Here's how the part is built. I have some questions about the finished solid (model axes, mm). Face numbers are marked on the shaded views. A direction names the side the tool comes from. Round coordinates to 2 decimals unless told otherwise and drop trailing zeros. Order: outer loops, then holes, each group sorted by start corner. A loop starts at its lowest first (then second) coordinate and runs counter-clockwise, first axis right, second up. Notation, with made-up numbers: (50.5, 39) -> (59.5, 39) arc R36 ccw to (59.5, 73) -> close; hole circle Ø6 at (83.5, 54.25). An arc over 180 degrees is marked (long way). Use a Markdown table: item, result. Add a question column.
(1) I want a section at D-D, the plane z = -23. Please give me the cut outline in (x, y), then the cut area to 3 significant figures.
(2) If I drill on probe 1 along X at (y, z) = (23.4, -13.5); probe 2 along Z at (x, y) = (15, 23); probe 3 along Z at (x, y) = (-26, 9), over which ranges is the centre line in solid material (lowest first)?
(3) I want a section at C-C, the plane z = -44.5. Please give me the cut outline in (x, y), then the cut area to 3 significant figures.
(4) I'm going to push flat-ended pins straight in: P1, Ø3, axis at x = 32, z = 0, coming from the +Y side; P2, Ø6.5, axis at x = 15.5, z = -45.5, coming from the -Y side; P3, Ø8, axis at y = 11.5, z = 2, coming from the -X side; P4, Ø12, axis at x = -1.5, z = -29, coming from the +Y side. Where does each tip first touch, or does it pass through?
(5) I want a section at B-B, the plane z = -29. Please give me the cut outline in (x, y).
(6) I want a section at A-A, the plane x = 0. Please give me the cut outline in (y, z).
(7) On a 3-axis mill with a long thin cutter (end or side, diameter ignored), from which of +Z, -Z, +X, -X, +Y, -Y can I reach the whole of each face in a straight line? I mean the marked faces 1, 2 and 3. Say none if no direction works.
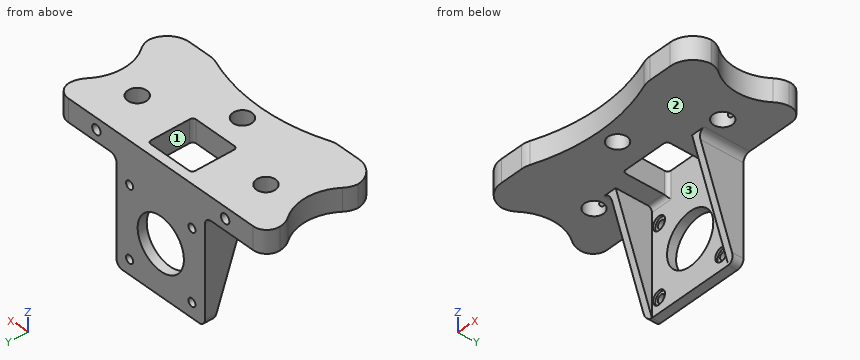
from build123d import *

# Parameters (mm, degrees)
SKETCH1_R           = 4.2
BOSS_EXTRUDE1_DEPTH = 5
FILLET1_R           = 10
FILLET2_R           = 6
SKETCH2_W           = 42
SKETCH2_H           = 46
SKETCH2_R           = 11.5
SKETCH2_R_2         = 1.75
BOSS_EXTRUDE2_DEPTH = 4
CUT_EXTRUDE1_REACH  = 89.139
CUT_EXTRUDE1_START  = -1
SKETCH3_R           = 3
CUT_EXTRUDE2_REACH  = 90.34
SKETCH4_R           = 1.75
SKETCH5_R           = 2.1
CUT_EXTRUDE3_DEPTH  = 4
CHAMFER1_SIZE       = 0.5
BOSS_EXTRUDE3_START = -2
BOSS_EXTRUDE3_DEPTH = 3
FILLET3_R           = 2
FILLET4_R           = 3


with BuildPart() as part:
    # Sketch1 → Boss-Extrude1 (new, symmetric)
    with BuildSketch(Plane.XY):
        with BuildLine():
            Line((-52, 25), (52, 25))
            Line((52, 25), (52, 15.565713714))
            ThreePointArc((52, 15.565713714), (46, 1.282856857), (52, -13))
            Line((52, -13), (52, -25))
            Line((52, -25), (30, -25))
            ThreePointArc((30, -25), (0, -19.161984871), (-30, -25))
            Line((-30, -25), (-52, -25))
            Line((-52, -25), (-52, -13))
            ThreePointArc((-52, -13), (-46, 1.282856857), (-52, 15.565713714))
            Line((-52, 15.565713714), (-52, 25))
        make_face()
        with Locations((0, -11)):
            Circle(SKETCH1_R, mode=Mode.SUBTRACT)
        with Locations((-32, 7)):
            Circle(SKETCH1_R, mode=Mode.SUBTRACT)
        with Locations((32, 7)):
            Circle(SKETCH1_R, mode=Mode.SUBTRACT)
        with BuildLine():
            Line((-9.5, 21), (9.5, 21))
            ThreePointArc((9.5, 21), (10.560660172, 20.560660172), (11, 19.5))
            Line((11, 19.5), (11, 2.5))
            ThreePointArc((11, 2.5), (10.560660172, 1.439339828), (9.5, 1))
            Line((9.5, 1), (-9.5, 1))
            ThreePointArc((-9.5, 1), (-10.560660172, 1.439339828), (-11, 2.5))
            Line((-11, 2.5), (-11, 19.5))
            ThreePointArc((-11, 19.5), (-10.560660172, 20.560660172), (-9.5, 21))
        make_face(mode=Mode.SUBTRACT)
    extrude(amount=BOSS_EXTRUDE1_DEPTH, both=True)

    # Fillet1
    # the kernel refuses this fillet: 10 mm, written as the material it takes off along each edge
    with BuildSketch(Plane(origin=(52, 15.565713714, 14.292857857), x_dir=(-0.6589710561597435, -0.7521682970876347, 0), z_dir=(0, 0, -1))) as fillet1_piece_1:
        with BuildLine():
            CenterArc((3.793793334, 9.971172714), FILLET1_R, 228.778553177, 36.869897646)
            Line((-2.795917228, 2.449489743), (0, 0))
            ThreePointArc((0, 0), (1.517517334, 0.057654573), (3.035034667, 0))
        make_face()
    extrude(amount=28.585715715, mode=Mode.SUBTRACT)
    with BuildSketch(Plane(origin=(52, -13, 14.292857857), x_dir=(0, -1, 0), z_dir=(0, 0, -1)), Plane(origin=(-52, -13, -14.292857857), x_dir=(0, -1, 0), z_dir=(0, 0, 1))) as fillet1_piece_2:
        with BuildLine():
            CenterArc((3.717143143, 10), FILLET1_R, 233.130102354, 36.869897646)
            ThreePointArc((-2.282856857, 2), (-1.103435734, 1.043365942), (0, 0))
            Line((0, 0), (3.717143143, 0))
        make_face()
    extrude(amount=28.585715715, mode=Mode.SUBTRACT)
    with BuildSketch(Plane(origin=(52, -25, 30), x_dir=(-1, 0, 0), z_dir=(0, 0, -1))) as fillet1_piece_3:
        with BuildLine():
            CenterArc((FILLET1_R, FILLET1_R), FILLET1_R, 180, 90)
            Line((0, FILLET1_R), (0, 0))
            Line((0, 0), (FILLET1_R, 0))
        make_face()
    extrude(amount=60, mode=Mode.SUBTRACT)
    with BuildSketch(Plane(origin=(30, -25, 9.716697693), x_dir=(-0.931136532102541, 0.3646707536724787, 0), z_dir=(0, 0, -1))) as fillet1_piece_4:
        with BuildLine():
            CenterArc((1.889951723, 9.999382002), FILLET1_R, 248.612678269, 20.750330625)
            Line((-1.756755813, 0.688016681), (0, 0))
            ThreePointArc((0, 0), (0.889389046, 0.004943983), (1.778778093, 0))
        make_face()
    extrude(amount=19.433395387, mode=Mode.SUBTRACT)
    with BuildSketch(Plane(origin=(-30, -25, 9.716697693), x_dir=(-1, 0, 0), z_dir=(0, 0, -1))) as fillet1_piece_5:
        with BuildLine():
            CenterArc((1.886679077, 10), FILLET1_R, 249.249669375, 20.750330625)
            ThreePointArc((-1.656285265, 0.648668348), (-0.826339706, 0.328937697), (0, 0))
            Line((0, 0), (1.886679077, 0))
        make_face()
    extrude(amount=19.433395387, mode=Mode.SUBTRACT)
    with BuildSketch(Plane(origin=(-52, -25, -30), x_dir=(0, 1, 0), z_dir=(0, 0, 1))) as fillet1_piece_6:
        with BuildLine():
            CenterArc((FILLET1_R, -FILLET1_R), FILLET1_R, 90, 90)
            Line((0, -FILLET1_R), (0, 0))
            Line((0, 0), (FILLET1_R, 0))
        make_face()
    extrude(amount=60, mode=Mode.SUBTRACT)
    with BuildSketch(Plane(origin=(-52, 15.565713714, -14.292857857), x_dir=(0, 1, 0), z_dir=(0, 0, 1))) as fillet1_piece_7:
        with BuildLine():
            CenterArc((3.717143143, -10), FILLET1_R, 90, 36.869897646)
            ThreePointArc((-2.282856857, -2), (-1.103435734, -1.043365942), (0, 0))
            Line((0, 0), (3.717143143, 0))
        make_face()
    extrude(amount=28.585715715, mode=Mode.SUBTRACT)

    # Fillet2
    fillet2_edges = [part.edges().sort_by_distance(p)[0] for p in [
        (52, 25, 0),
        (-52, 25, 0),
    ]]
    fillet(fillet2_edges, radius=FILLET2_R)

    # Sketch2 → Boss-Extrude2 (add)
    with BuildSketch(Plane(origin=(0, 25, -30), x_dir=(-1, 0, 0), z_dir=(0, 1, 0))):
        with Locations((0, 2)):
            Rectangle(SKETCH2_W, SKETCH2_H)
        with Locations(Location((0, 1, 0), (0, 0, 90))):
            Circle(SKETCH2_R, mode=Mode.SUBTRACT)
        with Locations(Location((15.5, 16.5, 0), (0, 0, 90))):
            Circle(SKETCH2_R_2, mode=Mode.SUBTRACT)
        with Locations(Location((-15.5, 16.5, 0), (0, 0, 90))):
            Circle(SKETCH2_R_2, mode=Mode.SUBTRACT)
        with Locations(Location((-15.5, -14.5, 0), (0, 0, 90))):
            Circle(SKETCH2_R_2, mode=Mode.SUBTRACT)
        with Locations(Location((15.5, -14.5, 0), (0, 0, 90))):
            Circle(SKETCH2_R_2, mode=Mode.SUBTRACT)
    extrude(amount=-BOSS_EXTRUDE2_DEPTH)

    # Sketch3 → Cut-Extrude1 (cut, up to next)
    with BuildSketch(Plane.XZ.offset(-21).offset(CUT_EXTRUDE1_START), mode=Mode.PRIVATE) as cut_extrude1_sk1:
        with Locations(Location((-15.5, -44.5, 0), (0, 0, 270))):
            Circle(SKETCH3_R)
    cut_extrude1_tool1 = extrude(cut_extrude1_sk1.sketch, amount=CUT_EXTRUDE1_REACH, mode=Mode.PRIVATE) & part.part
    # Sketch3 → Cut-Extrude1 (cut, up to next)
    with BuildSketch(Plane.XZ.offset(-21).offset(CUT_EXTRUDE1_START), mode=Mode.PRIVATE) as cut_extrude1_sk2:
        with Locations(Location((15.5, -44.5, 0), (0, 0, 270))):
            Circle(SKETCH3_R)
    cut_extrude1_tool2 = extrude(cut_extrude1_sk2.sketch, amount=CUT_EXTRUDE1_REACH, mode=Mode.PRIVATE) & part.part
    # Sketch3 → Cut-Extrude1 (cut, up to next)
    with BuildSketch(Plane.XZ.offset(-21).offset(CUT_EXTRUDE1_START), mode=Mode.PRIVATE) as cut_extrude1_sk3:
        with Locations(Location((15.5, -13.5, 0), (0, 0, 270))):
            Circle(SKETCH3_R)
    cut_extrude1_tool3 = extrude(cut_extrude1_sk3.sketch, amount=CUT_EXTRUDE1_REACH, mode=Mode.PRIVATE) & part.part
    # Sketch3 → Cut-Extrude1 (cut, up to next)
    with BuildSketch(Plane.XZ.offset(-21).offset(CUT_EXTRUDE1_START), mode=Mode.PRIVATE) as cut_extrude1_sk4:
        with Locations(Location((-15.5, -13.5, 0), (0, 0, 270))):
            Circle(SKETCH3_R)
    cut_extrude1_tool4 = extrude(cut_extrude1_sk4.sketch, amount=CUT_EXTRUDE1_REACH, mode=Mode.PRIVATE) & part.part
    add(cut_extrude1_tool1.solids().sort_by_distance((-15.5, 22, -44.5))[0], mode=Mode.SUBTRACT)
    add(cut_extrude1_tool2.solids().sort_by_distance((15.5, 22, -44.5))[0], mode=Mode.SUBTRACT)
    add(cut_extrude1_tool3.solids().sort_by_distance((15.5, 22, -13.5))[0], mode=Mode.SUBTRACT)
    add(cut_extrude1_tool4.solids().sort_by_distance((-15.5, 22, -13.5))[0], mode=Mode.SUBTRACT)

    # Sketch4 → Cut-Extrude2 (cut, up to next)
    with BuildSketch(Plane(origin=(0, 25, 0), x_dir=(1, 0, 0), z_dir=(0, 1, 0)), mode=Mode.PRIVATE) as cut_extrude2_sk1:
        with Locations(Location((-32, 0, 0), (0, 0, 270))):
            Circle(SKETCH4_R)
    cut_extrude2_tool1 = extrude(cut_extrude2_sk1.sketch, amount=-CUT_EXTRUDE2_REACH, mode=Mode.PRIVATE) & part.part
    # Sketch4 → Cut-Extrude2 (cut, up to next)
    with BuildSketch(Plane(origin=(0, 25, 0), x_dir=(1, 0, 0), z_dir=(0, 1, 0)), mode=Mode.PRIVATE) as cut_extrude2_sk2:
        with Locations(Location((32, 0, 0), (0, 0, 270))):
            Circle(SKETCH4_R)
    cut_extrude2_tool2 = extrude(cut_extrude2_sk2.sketch, amount=-CUT_EXTRUDE2_REACH, mode=Mode.PRIVATE) & part.part
    add(cut_extrude2_tool1.solids().sort_by_distance((-32, 25, 0))[0], mode=Mode.SUBTRACT)
    add(cut_extrude2_tool2.solids().sort_by_distance((32, 25, 0))[0], mode=Mode.SUBTRACT)

    # Sketch5 → Cut-Extrude3 (cut)
    with BuildSketch(Plane(origin=(0, 25, 0), x_dir=(1, 0, 0), z_dir=(0, 1, 0))):
        with Locations(Location((-32, 0, 0), (0, 0, 270))):
            Circle(SKETCH5_R)
        with Locations(Location((32, 0, 0), (0, 0, 270))):
            Circle(SKETCH5_R)
    extrude(amount=-CUT_EXTRUDE3_DEPTH, mode=Mode.SUBTRACT)

    # Chamfer1
    # the kernel refuses this chamfer: 0.5 mm, written as the material it adds along each edge
    # the kernel refuses this chamfer: 0.5 mm, written as the material it takes off along each edge
    with BuildSketch(Plane(origin=(-32, 21, 0), x_dir=(0, 0, 1), z_dir=(-1, 0, 0))) as chamfer1_2_piece_1_section:
        Polygon((1.75, -CHAMFER1_SIZE), (1.75 + CHAMFER1_SIZE, 0), (1.75, 0), align=None)
    chamfer1_2_piece_1 = revolve(axis=Axis((-32, 21, 0), (0, 1, 0)), mode=Mode.PRIVATE)
    chamfer1_2_piece_1 = chamfer1_2_piece_1 & Plane(origin=(-32, 20.682821512, 0), x_dir=(0, 0, 1), z_dir=(0, 1, 0)) * Cylinder(2.1, 9, mode=Mode.PRIVATE)
    add(chamfer1_2_piece_1, mode=Mode.SUBTRACT)
    with BuildSketch(Plane(origin=(32, 21, 0), x_dir=(0, 0, 1), z_dir=(-1, 0, 0))) as chamfer1_2_piece_2_section:
        Polygon((1.75, -CHAMFER1_SIZE), (1.75 + CHAMFER1_SIZE, 0), (1.75, 0), align=None)
    chamfer1_2_piece_2 = revolve(axis=Axis((32, 21, 0), (0, 1, 0)), mode=Mode.PRIVATE)
    chamfer1_2_piece_2 = chamfer1_2_piece_2 & Plane(origin=(32, 20.682821512, 0), x_dir=(0, 0, 1), z_dir=(0, 1, 0)) * Cylinder(2.1, 10, mode=Mode.PRIVATE)
    add(chamfer1_2_piece_2, mode=Mode.SUBTRACT)

    # Sketch6 → Boss-Extrude3 (add)
    with BuildSketch(Plane.ZY.offset(21).offset(BOSS_EXTRUDE3_START)):
        Polygon((-51, 25), (-5, 25), (-5, 5), (-51, 21), align=None)
    boss_extrude3 = extrude(amount=BOSS_EXTRUDE3_DEPTH)

    # Mirror1: Boss-Extrude3 across plane
    add(boss_extrude3.mirror(Plane(origin=(0, 0, 0), x_dir=(0, 0, 1), z_dir=(1, 0, 0))))

    # Fillet3
    fillet3_edges = [part.edges().sort_by_distance(p)[0] for p in [
        (-14.25, 21, -5),
        (14.25, 21, -5),
    ]]
    fillet(fillet3_edges, radius=FILLET3_R)

    # Fillet4
    fillet4_edges = [part.edges().sort_by_distance(p)[0] for p in [
        (-22, 23, -51),
        (22, 23, -51),
        (-22, 15, -5),
        (22, 15, -5),
    ]]
    fillet(fillet4_edges, radius=FILLET4_R)


solid = part.part
Taken from the geometry:
| question | item | result |
|---|---|---|
| 1 | outline | (-22, 11.26) -> (-19, 11.26) -> (-19, 21) -> (-9.81, 21) -> (-9.81, 25) -> (-22, 25) -> close; (9.81, 21) -> (19, 21) -> (19, 11.26) -> (22, 11.26) -> (22, 25) -> (9.81, 25) -> close |
| 1 | area | 156 mm2 |
| 2 | probe 1 | x = -22 to -17.25, -13.75 to 13.75, 17.25 to 22 |
| 2 | probe 2 | z = -51 to -46.18, -42.82 to -15.18, -11.82 to 5 |
| 2 | probe 3 | z = -5 to 5 |
| 3 | outline | (-22, 18.74) -> (-19, 18.74) -> (-19, 21) -> (-18.5, 21) -> (-18.5, 22) -> (-17.25, 22) -> (-17.25, 25) -> (-22, 25) -> close; (-13.75, 22) -> (-12.5, 22) -> (-12.5, 21) -> (12.5, 21) -> (12.5, 22) -> (13.75, 22) -> (13.75, 25) -> (-13.75, 25) -> close; (17.25, 22) -> (18.5, 22) -> (18.5, 21) -> (19, 21) -> (19, 18.74) -> (22, 18.74) -> (22, 25) -> (17.25, 25) -> close |
| 3 | area | 157 mm2 |
| 4 | P1 | stops at y = 3.08 |
| 4 | P2 | stops at y = 21 |
| 4 | P3 | stops at x = -51.26 |
| 4 | P4 | passes through |
| 5 | outline | (-22, 13.35) -> (-19, 13.35) -> (-19, 21) -> (-11.5, 21) -> (-11.5, 25) -> (-22, 25) -> close; (11.5, 21) -> (19, 21) -> (19, 13.35) -> (22, 13.35) -> (22, 25) -> (11.5, 25) -> close |
| 6 | outline | (-19.16, -5) -> (-15.2, -5) -> (-15.2, 5) -> (-19.16, 5) -> close; (-6.8, -5) -> (1, -5) -> (1, 5) -> (-6.8, 5) -> close; (21, -51) -> (25, -51) -> (25, -40.5) -> (21, -40.5) -> close; (21, -17.5) -> (25, -17.5) -> (25, 5) -> (21, 5) -> close |
| 7 | face 1 | +Z, -Z |
| 7 | face 2 | -Z, -Y |
| 7 | face 3 | -Z |
